```python
from build123d import *

# Parameters (mm, degrees)
BOSS_EXTRUDE1_DEPTH            = 4.7625
BOSS_EXTRUDE1_DEPTH_BACK       = 1.651
SKETCH1_W                      = 63.5
SKETCH1_H                      = 190.5
SKETCH3_R                      = 6.35
CUT_EXTRUDE1_DEPTH             = 0.508
SKETCH4_R                      = 18.25625
BOSS_EXTRUDE2_DEPTH            = 38.1
SKETCH5_R                      = 12.461875
CUT_EXTRUDE2_DEPTH             = 38.1
SKETCH7_R                      = 14.2875
CUT_EXTRUDE3_DEPTH             = 30.48
F_3_16_0_1875_DIAMETER_HOLE1_D = 4.7625
SKETCH13_R                     = 14.478
CUT_EXTRUDE4_DEPTH             = 30.48
CUT_EXTRUDE5_START             = -12.7
SKETCH14_R                     = 18.25625
CUT_EXTRUDE5_DEPTH             = 12.7
F_3_16_0_1875_DIAMETER_HOLE3_D = 4.7625


with BuildPart() as part:
    # Sketch1 → Boss-Extrude1 (new, two sides: drawn at the far end of the back side and taken through both)
    with BuildSketch(Plane.XY.offset(-BOSS_EXTRUDE1_DEPTH_BACK)):
        Rectangle(SKETCH1_W, SKETCH1_H)
    extrude(amount=BOSS_EXTRUDE1_DEPTH + BOSS_EXTRUDE1_DEPTH_BACK)

    # Sketch3 → Cut-Extrude1 (cut)
    with BuildSketch(Plane.XY.offset(4.7625)):
        Circle(SKETCH3_R)
    extrude(amount=-CUT_EXTRUDE1_DEPTH, mode=Mode.SUBTRACT)

    # Sketch4 → Boss-Extrude2 (add)
    with BuildSketch(Plane.XY.offset(4.7625)):
        with Locations(Location((0, 0, 0), (0, 0, 180))):
            Circle(SKETCH4_R)
    extrude(amount=BOSS_EXTRUDE2_DEPTH)

    # Sketch5 → Cut-Extrude2 (cut)
    with BuildSketch(Plane.XY.offset(42.8625)):
        Circle(SKETCH5_R)
    extrude(amount=-CUT_EXTRUDE2_DEPTH, mode=Mode.SUBTRACT)

    # Sketch7 → Cut-Extrude3 (cut)
    with BuildSketch(Plane.XY.offset(42.8625)):
        Circle(SKETCH7_R)
    extrude(amount=-CUT_EXTRUDE3_DEPTH, mode=Mode.SUBTRACT)

    # 3/16 (0.1875) Diameter Hole1 (through all)
    with Locations(Plane.XY.offset(4.7625)):
        with Locations((-22.225, 85.725), (-22.225, -85.725), (22.225, -85.725), (22.225, 85.725), (0, 48.514), (0, -48.514), (-22.225, 22.225), (-22.225, -22.225), (22.225, -22.225), (22.225, 22.225)):
            Hole(F_3_16_0_1875_DIAMETER_HOLE1_D / 2)

    # Sketch13 → Cut-Extrude4 (cut)
    with BuildSketch(Plane.XY.offset(42.8625)):
        Circle(SKETCH13_R)
    extrude(amount=-CUT_EXTRUDE4_DEPTH, mode=Mode.SUBTRACT)

    # Sketch14 → Cut-Extrude5 (cut)
    with BuildSketch(Plane.XY.offset(42.8625).offset(CUT_EXTRUDE5_START)):
        with Locations(Location((0, 0, 0), (0, 0, 180))):
            Circle(SKETCH14_R)
    extrude(amount=CUT_EXTRUDE5_DEPTH, mode=Mode.SUBTRACT)

    # 3/16 (0.1875) Diameter Hole3 (through all)
    with Locations(Plane(origin=(18.25625, 0, 21.873504095), x_dir=(0, 1, 0), z_dir=(1, 0, 0))):
        with Locations((0, 0)):
            Hole(F_3_16_0_1875_DIAMETER_HOLE3_D / 2)


solid = part.part
```
Here's how the part is built. I have some questions about the finished solid (model axes, mm). A direction names the side the tool comes from. Round coordinates to 2 decimals unless told otherwise and drop trailing zeros. Order: outer loops, then holes, each group sorted by start corner. A loop starts at its lowest first (then second) coordinate and runs counter-clockwise, first axis right, second up. Notation, with made-up numbers: M 16,81.5 L 60,81.5 A34 cw 60,118.5 Z; hole C -5.75,25.25 d11. An arc over 180 degrees is marked long. Use CSV: the item, a comma, the result in double quotes.
1) On a 3-axis mill with a long thin cutter (end or side, diameter ignored), from which of +Z, -Z, +X, -X, +Y, -Y can I reach the whole of each face in a straight line? I mean faces 5 (the cylindrical face through (-21.71, 19.9, 1.51)), 6 (the flat face through (0, 0, 4.254)). Say none if no direction works.
Taken from the geometry:
face 5,"+Z, -Z"
face 6,"+Z"
2) If we mould it in two halves opening along Y, with no side actions, what happens to faces 1 (the flat face through (0, 95.25, 2)), 2 (the cylindrical face through (-17.413, -5.484, 17.285)), 3 (the flat face through (0, -95.25, 2)), 4 (the flat face through (4, 12, 12.382))? For each: pulls with the +Y half, pulls with the -Y half, needs draft (parallel to the pull), parting line crosses it, or undercut.
Taken from the geometry:
face 1,"pulls with the +Y half"
face 2,"parting line crosses it"
face 3,"pulls with the -Y half"
face 4,"undercut"
3) I need wall thicknesses on line 1 along Y through (x, z) = (0, 1); line 2 along Z through (x, y) = (-7, 45.5); line 3 along Y through (x, z) = (-9.5, 11). Which ranges of each line are inside material? Lowest first, please. Write a range as [from, to].
Taken from the geometry:
line 1,"[-95.25, -50.9], [-46.13, 46.13], [50.9, 95.25]"
line 2,"[-1.65, 4.76]"
line 3,"[-15.59, -8.07], [8.07, 15.59]"
4) I want a section at C-C (z = 7.5). List the corners of the cut face in (x, y) for me, then the cut area to 3 significant figures.
Taken from the geometry:
outline,"C 0,0 d36.51; hole C 0,0 d24.92"
area,"559 mm^2"
5) I want a section at A-A (x = 0). List the corners of the cut face in (y, z) for me.
Taken from the geometry:
outline,"M -95.25,-1.65 L -50.9,-1.65 L -50.9,4.76 L -95.25,4.76 Z; M -46.13,-1.65 L 46.13,-1.65 L 46.13,4.76 L 18.26,4.76 L 18.26,30.16 L 14.48,30.16 L 14.48,12.38 L 12.46,12.38 L 12.46,4.76 L 6.35,4.76 L 6.35,4.25 L -6.35,4.25 L -6.35,4.76 L -12.46,4.76 L -12.46,12.38 L -14.48,12.38 L -14.48,30.16 L -18.26,30.16 L -18.26,4.76 L -46.13,4.76 Z; M 50.9,-1.65 L 95.25,-1.65 L 95.25,4.76 L 50.9,4.76 Z"
6) I'm going to push flat-ended pins straight in: P1, Ø4, axis at x = -17.5, z = 25, coming from the -Y side; P2, Ø5.5, axis at y = 0, z = 21.87, coming from the +X side; P3, Ø20, axis at x = 0, y = 0, coming from the +Z side. Where does each tip first touch, or does it pass through?
Taken from the geometry:
P1,"y = -9.65"
P2,"x = 18.26"
P3,"z = 4.76"
7) I want a section at B-B (y = 0). List the corners of the cut face in (x, z) for me, then the cut area to 3 significant figures.
Taken from the geometry:
outline,"M -31.75,-1.65 L 31.75,-1.65 L 31.75,4.76 L 18.26,4.76 L 18.26,19.49 L 14.48,19.49 L 14.48,12.38 L 12.46,12.38 L 12.46,4.76 L 6.35,4.76 L 6.35,4.25 L -6.35,4.25 L -6.35,4.76 L -12.46,4.76 L -12.46,12.38 L -14.48,12.38 L -14.48,19.49 L -18.26,19.49 L -18.26,4.76 L -31.75,4.76 Z; M -18.26,24.25 L -14.48,24.25 L -14.48,30.16 L -18.26,30.16 Z; M 14.48,24.25 L 18.26,24.25 L 18.26,30.16 L 14.48,30.16 Z"
area,"587 mm^2"
8) I want a section at D-D (y = 36). List the corners of the cut face in (x, z) for me, then the cut area to 3 significant figures.
Taken from the geometry:
outline,"M -31.75,-1.65 L 31.75,-1.65 L 31.75,4.76 L -31.75,4.76 Z"
area,"407 mm^2"
